Geometry check sheet. Reference: the model listing, model coordinates, mm. A direction names the side the tool comes from. Give positions to 0.01 mm unless a question says otherwise; leave off trailing zeros. Order: outer loops, then holes, each group sorted by start corner. A loop starts at its lowest first (then second) coordinate and runs counter-clockwise, first axis right, second up. Notation, with made-up numbers: M -37.75,-24.5 L -12.75,-24.5 A32 cw -12.75,7.5 Z; hole C -11.5,62 d5. An arc over 180 degrees is marked long. One line per question, with ' | ' between items. Start each with the question number.
from build123d import *

# Parameters (mm, degrees)
F0_R     = 1.8
F0_W     = 14
F0_H     = 14
F1_DEPTH = 4
F0_H_2   = 4
F2_DEPTH = 20
F3_R     = 5
F4_DEPTH = 4
F5_SIZE  = 1.5


with BuildPart() as f1:
    # F0 (on Top) → F1 (new body)
    with BuildSketch(Plane.XY):
        Polygon((0, 6), (-30, 6), (-30, 0), (-22, 0), (-8, 0), (0, 0), align=None)
        with Locations((-26, 3)):
            Circle(F0_R, mode=Mode.SUBTRACT)
        with Locations((-4, 3)):
            Circle(F0_R, mode=Mode.SUBTRACT)
        with Locations((-15, -7)):
            Rectangle(F0_W, F0_H)
    extrude(amount=F1_DEPTH)

    # F0 (on Top) → F2 (join)
    with BuildSketch(Plane.XY):
        with Locations((-15, -16)):
            Rectangle(F0_W, F0_H_2)
    extrude(amount=F2_DEPTH)

    # F3 (on face) → F4 (cut, through all)
    with BuildSketch(Plane(origin=(0, -14, 0), x_dir=(-1, 0, 0), z_dir=(0, 1, 0))):
        with Locations((15, 13)):
            Circle(F3_R)
    extrude(amount=-F4_DEPTH, mode=Mode.SUBTRACT)

    # F5
    f5_edges = [f1.edges().sort_by_distance(p)[0] for p in [
        (-15, -14, 4),
        (-22, -16, 20),
        (-8, -16, 20),
        (-22, 0, 2),
        (-8, 0, 2),
    ]]
    chamfer(f5_edges, length=F5_SIZE)


solid = f1.part
Item 1: Depth check by flat-ended pin: pin 1 (4.5 mm diameter, centred on x = -26.5, z = 2.5, fed in from -Y); pin 2 (8 mm diameter, centred on y = -12.5, z = 3, fed in from +X); pin 3 (3 mm diameter, centred on x = -13, z = 8.5, fed in from +Y); pin 4 (9 mm diameter, centred on x = -15, z = 13, fed in from +Y). Enter the tip coordinate at first touch or a pass-through.
Item 2: Material ranges on line 1 along Z through (x, y) = (-15, -15.65); line 2 along Y through (x, z) = (-26, 1.6); line 3 along Y through (x, z) = (-20.25, 17.75), recorded low to high.
Item 3: Cross-section at B-B, the plane z = 3.25. Record the cut outline in (x, y), plus the area to 3 significant figures.
Item 4: Set-up check for faces 1 (the flat face through (-8, -14, 5)), 2 (the flat face through (-15, -1, 4)), 3 (the flat face through (-22, -14, 5)): record each of +Z, -Z, +X, -X, +Y, -Y from which the full face is reachable in a straight line by a thin tool's end or side.
Item 5: Cross-section at A-A, the plane y = 3. Record the cut outline in (x, z), plus the area to 3 significant figures.
Item 6: Mould release check, pull along X, two halves, no side actions. Record for faces 4 (the flat face through (0, 3, 2)), 5 (the cylindrical face through (-3.032, 4.518, 1.972)), 6 (the flat face through (-27, 0, 2)): released by +X, released by -X, zero draft, split by the parting line, or undercut.
Item 7: Cross-section at C-C, the plane x = -3.25. Record the cut outline in (y, z).
Item 8: Cross-section at D-D, the plane z = 14.25. Record the cut outline in (x, y), plus the area to 3 significant figures.
Outcome:
1) pin 1: stops at y = 0 | pin 2: stops at x = -8 | pin 3: stops at y = -14 | pin 4: passes through
2) line 1: z = 0 to 8, 18 to 20 | line 2: y = 0 to 1.2, 4.8 to 6 | line 3: y = -18 to -14
3) outline: M -30,0 L -23.5,0 L -22,-1.5 L -22,-18 L -8,-18 L -8,-1.5 L -6.5,0 L 0,0 L 0,6 L -30,6 Z; hole C -26,3 d3.6; hole C -4,3 d3.6 | area: 414 mm²
4) face 1: +Z, -Z, +X, -Y | face 2: +Z, +X, -X, +Y | face 3: +Z, -Z, -X, -Y
5) outline: M -30,0 L -27.8,0 L -27.8,4 L -30,4 Z; M -24.2,0 L -5.8,0 L -5.8,4 L -24.2,4 Z; M -2.2,0 L 0,0 L 0,4 L -2.2,4 Z | area: 91.2 mm²
6) face 4: released by +X | face 5: undercut | face 6: zero draft
7) outline: M 0,0 L 1.36,0 L 1.36,4 L 0,4 Z; M 4.64,0 L 6,0 L 6,4 L 4.64,4 Z
8) outline: M -22,-18 L -19.84,-18 L -19.84,-14 L -22,-14 Z; M -10.16,-18 L -8,-18 L -8,-14 L -10.16,-14 Z | area: 17.3 mm²
